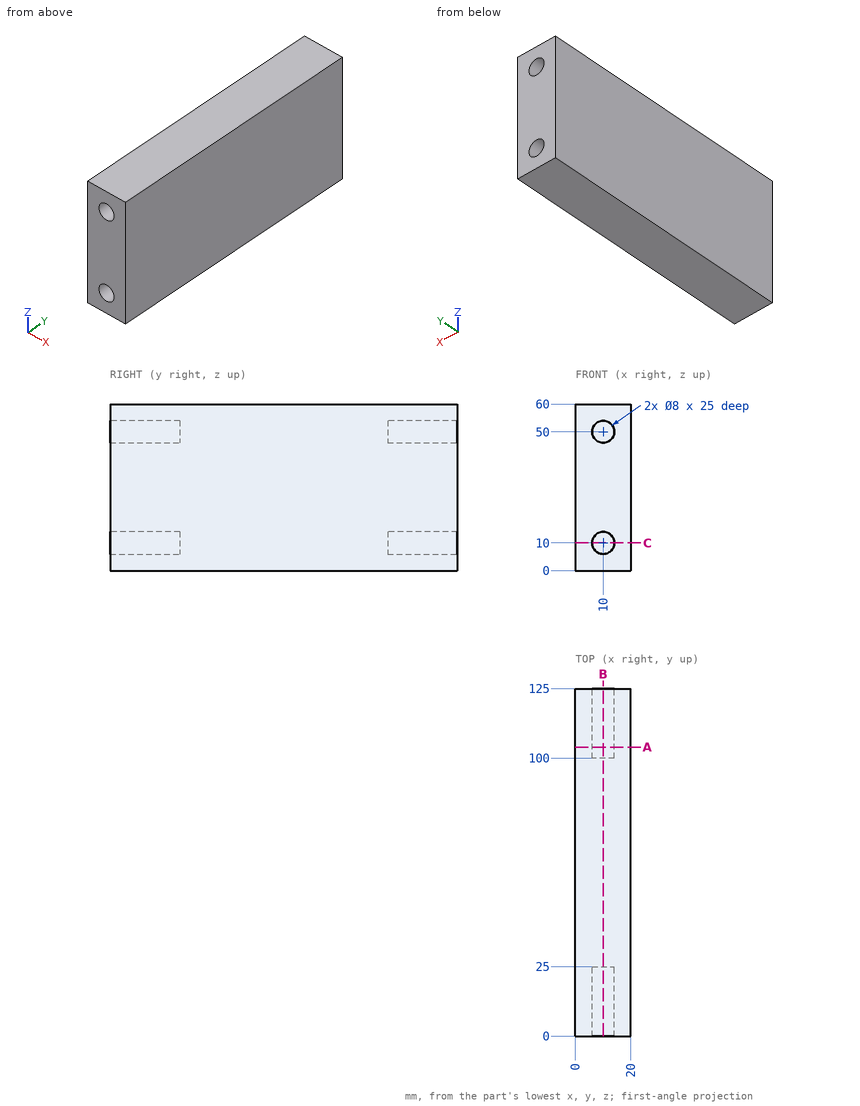
Here's the drawing with two shaded views (mm, measured from the low corner). I have some questions. Coordinates: 2 decimals unless noted, no trailing zeros. Loops run counter-clockwise (first coordinate to the right, second up) from the corner with the lowest first, then second, coordinate; pieces in that order, holes last.
Item 1: Suppose I cut it at B-B (x = 10). Please give me the cut outline in (y, z).
Answers below:
outline: (0, 0) - (125, 0) - (125, 6) - (100, 6) - (100, 14) - (125, 14) - (125, 46) - (100, 46) - (100, 54) - (125, 54) - (125, 60) - (0, 60) - (0, 54) - (25, 54) - (25, 46) - (0, 46) - (0, 14) - (25, 14) - (25, 6) - (0, 6) - close
Item 2: Suppose I cut it at C-C (z = 10). Please give me the cut outline in (x, y).
Answers below:
outline: (0, 0) - (6, 0) - (6, 25) - (14, 25) - (14, 0) - (20, 0) - (20, 125) - (14, 125) - (14, 100) - (6, 100) - (6, 125) - (0, 125) - close
Item 3: I'm going to push flat-ended pins straight in: pin 1 (4 mm diameter, centred on x = 9.5, z = 51.5, fed in from +Y); pin 2 (5 mm diameter, centred on x = 10, z = 50, fed in from -Y); pin 3 (1 mm diameter, centred on y = 58, z = 50.5, fed in from -X). Where does each tip first touch, or does it pass through?
Answers below:
pin 1: stops at y = 100
pin 2: stops at y = 25
pin 3: stops at x = 0
Item 4: Suppose I cut it at A-A (y = 104). Please give me the cut outline in (x, z).
Answers below:
outline: (0, 0) - (20, 0) - (20, 60) - (0, 60) - close; hole circle Ø8 at (10, 10); hole circle Ø8 at (10, 50)
Item 5: Please list where these lines run through material, in increasing order: L1, parallel to Z at x = 10, y = 7.25; L2, parallel to Z at x = 8.25, y = 13; L3, parallel to Y at x = 10, z = 9.
Answers below:
L1: z = 0 to 6, 14 to 46, 54 to 60
L2: z = 0 to 6.4, 13.6 to 46.4, 53.6 to 60
L3: y = 25 to 100
